Source: CAD feature listing. Evaluate the final solid. Frame: model axes, mm. Face numbers are marked on the shaded views. A direction names the side the tool comes from. Round coordinates to 2 decimals unless told otherwise and drop trailing zeros. Write each loop counter-clockwise with the first axis right and the second up, starting at its lowest first coordinate (ties: lowest second). Pieces come first, ordered by that corner, then holes. Notation, with made-up numbers: M -37.75,82.25 L 1.25,82.25 A21 cw 1.25,96.25 Z; hole C 43.5,-19 d3. An arc over 180 degrees is marked long. Answer in a Markdown table with one row per item. Add a question column.
Item 1: Cut plane B-B on x = 20. Return loops of the section in (y, z), and give its area (3 significant figures).
Item 2: Cut plane D-D on y = 10.5. Return loops of the section in (x, z).
Item 3: Contact query for flat-ended pins moving along their axis: pin 1 (5 mm diameter, centred on y = 5, z = 4, fed in from +X); pin 2 (5 mm diameter, centred on y = 7, z = 4, fed in from -X); pin 3 (2 mm diameter, centred on x = 1.5, z = -7.5, fed in from -Y); pin 4 (3 mm diameter, centred on x = -23.5, y = 7.5, fed in from -Z). Output: stop coordinate, or through.
Item 4: Set-up query: the marked faces 1, 2 and 3. Return all of +Z, -Z, +X, -X, +Y, -Y with unobstructed straight access to the full face (end or side cutting, diameter ignored); none if empty.
Item 5: Material intervals for probe 1 along X at (y, z) = (6.35, 19.75) (3 decimals); probe 2 along Y at (x, z) = (-19, 19); probe 3 along X at (y, z) = (2.75, 0), sorted ascending.
Item 6: Cut plane C-C on z = 5. Return loops of the section in (x, y), and give its area (3 significant figures).
Item 7: Mould query, pull axis Z, two halves, no side actions, for the marked faces 4, 5, 6 and 7. Classes: released by +Z, released by -Z, zero draft, split by the parting line, or undercut.
Item 8: Cut plane A-A on y = 6.35. Return loops of the section in (x, z) (3 decimals), and give its area (3 significant figures).
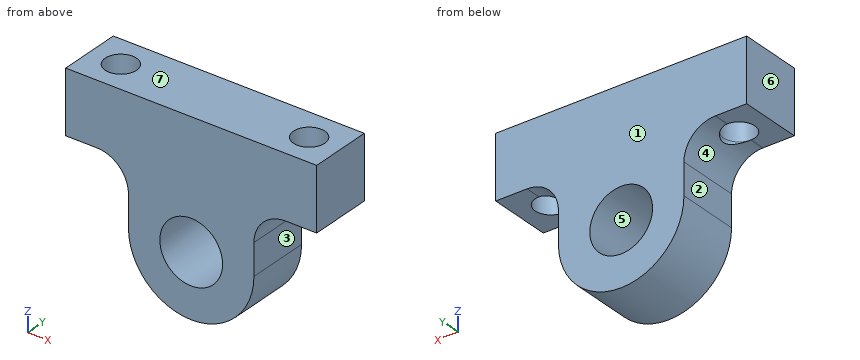
from build123d import *

# Parameters (mm, degrees)
SKETCH1_R               = 6.35
BOSS_EXTRUDE1_DEPTH     = 12.7
FILLET1_R               = 6.35
SKETCH2_R               = 3.175
CUT_EXTRUDE1_DEPTH      = 26.4
CUT_EXTRUDE1_DEPTH_BACK = 13.7


with BuildPart() as part:
    # Sketch1 → Boss-Extrude1 (new body)
    with BuildSketch(Plane(origin=(0, 0, 0), x_dir=(1, 0, 0), z_dir=(0, 1, 0))):
        with BuildLine():
            Line((-12.7, 0), (-12.7, -12.7))
            Line((-12.7, -12.7), (-25.4, -12.7))
            Line((-25.4, -12.7), (-25.4, -25.4))
            Line((-25.4, -25.4), (25.4, -25.4))
            Line((25.4, -25.4), (25.4, -12.7))
            Line((25.4, -12.7), (12.7, -12.7))
            Line((12.7, -12.7), (12.7, 0))
            ThreePointArc((12.7, 0), (0, 12.7), (-12.7, 0))
        make_face()
        Circle(SKETCH1_R, mode=Mode.SUBTRACT)
    extrude(amount=BOSS_EXTRUDE1_DEPTH)

    # Fillet1
    fillet1_edges = [part.edges().sort_by_distance(p)[0] for p in [
        (12.7, 6.35, 12.7),
        (-12.7, 6.35, 12.7),
    ]]
    fillet(fillet1_edges, radius=FILLET1_R)

    # Sketch2 → Cut-Extrude1 (cut, two sides)
    with BuildSketch(Plane(origin=(0, 0, 12.7), x_dir=(-1, 0, 0), z_dir=(0, 0, -1))) as cut_extrude1_sk:
        with Locations((19.05, 6.35)):
            Circle(SKETCH2_R)
        with Locations((-19.05, 6.35)):
            Circle(SKETCH2_R)
    extrude(amount=CUT_EXTRUDE1_DEPTH, mode=Mode.SUBTRACT)
    extrude(cut_extrude1_sk.sketch, amount=-CUT_EXTRUDE1_DEPTH_BACK, mode=Mode.SUBTRACT)


solid = part.part
Results below:
| question | item | result |
|---|---|---|
| 1 | outline | M 0,12.7 L 3.32,12.7 L 3.32,25.4 L 0,25.4 Z; M 9.38,12.7 L 12.7,12.7 L 12.7,25.4 L 9.38,25.4 Z |
| 1 | area | 84.3 mm2 |
| 2 | outline | M -25.4,12.7 L -19.05,12.7 A6.35 cw -12.7,6.35 L -12.7,0 A12.7 ccw 12.7,0 L 12.7,6.35 A6.35 cw 19.05,12.7 L 25.4,12.7 L 25.4,25.4 L -25.4,25.4 Z; hole C 0,0 d12.7 |
| 3 | pin 1 | x = 12.7 |
| 3 | pin 2 | x = -12.7 |
| 3 | pin 3 | y = 0 |
| 3 | pin 4 | z = 12.7 |
| 4 | face 1 | +Z, -Z, +X, -X, +Y |
| 4 | face 2 | -Z, -X, +Y, -Y |
| 4 | face 3 | -Z, +X, +Y, -Y |
| 5 | probe 1 | -25.4 to -22.225, -15.875 to 15.875, 22.225 to 25.4 |
| 5 | probe 2 | 0 to 3.18, 9.52 to 12.7 |
| 5 | probe 3 | -12.7 to -6.35, 6.35 to 12.7 |
| 6 | outline | M -12.7,0 L -3.91,0 L -3.91,12.7 L -12.7,12.7 Z; M 3.91,0 L 12.7,0 L 12.7,12.7 L 3.91,12.7 Z |
| 6 | area | 223 mm2 |
| 7 | face 4 | released by -Z |
| 7 | face 5 | undercut |
| 7 | face 6 | zero draft |
| 7 | face 7 | released by +Z |
| 8 | outline | M -25.4,12.7 L -22.225,12.7 L -22.225,25.4 L -25.4,25.4 Z; M -15.875,11.849 A6.35 cw -12.7,6.35 L -12.7,0 A12.7 ccw 12.7,0 L 12.7,6.35 A6.35 cw 15.875,11.849 L 15.875,25.4 L -15.875,25.4 Z; M 22.225,12.7 L 25.4,12.7 L 25.4,25.4 L 22.225,25.4 Z; hole C 0,0 d12.7 |
| 8 | area | 949 mm2 |
